Check sheet for the modelled part. Datum: model origin and axes. Units: mm. Face numbers are marked on the shaded views. Give positions to 0.01 mm unless a question says otherwise; leave off trailing zeros. Loops run counter-clockwise (first coordinate to the right, second up) from the corner with the lowest first, then second, coordinate; pieces in that order, holes last. Notation, with made-up numbers: M 14.25,83.5 L 54.25,83.5 A32 cw 54.25,117.5 Z; hole C 52,75 d4. An arc over 180 degrees is marked long. Write each question's results on one line, items separated by ' | '. Start each with the question number.
1. Material ranges on line 1 along X through (y, z) = (37, 0) (3 decimals); line 2 along Y through (x, z) = (-1.5, 22) (3 decimals); line 3 along Z through (x, y) = (-1.5, 36.5), recorded low to high.
2. Sectioned sample at C-C on y = 12. Record the cut outline in (x, z) (3 decimals).
3. Sectioned sample at A-A on z = 0. Record the cut outline in (x, y) (3 decimals), and give its area (3 significant figures).
4. Draft check along X on the marked faces 1, 2 and 3. Enter one of: pulls with the +X half, pulls with the -X half, needs draft (parallel to the pull), parting line crosses it, or undercut.
5. Go/stop test with flat-tipped pins: pin 1 (10 mm diameter, centred on x = -21.5, y = 41.5, fed in from +Z); pin 2 (1.5 mm diameter, centred on y = 16, z = 2.5, fed in from +X); pin 3 (12 mm diameter, centred on x = 23.5, z = -18.5, fed in from +Y); pin 4 (6 mm diameter, centred on y = 31, z = -3, fed in from -X). Record where each tip stops, or that it passes through.
6. Sectioned sample at B-B on x = 0. Record the cut outline in (y, z) (3 decimals), and give its area (3 significant figures).
```python
from build123d import *

# Parameters (mm, degrees)
SKETCH2_R           = 31.75
BOSS_EXTRUDE2_DEPTH = 50.8
SHELL1_T            = -3.175
FILLET2_R           = 2.54
CHAMFER1_SIZE       = 2.54


with BuildPart() as part:
    # Sketch2 → Boss-Extrude2 (new body)
    with BuildSketch(Plane(origin=(0, 0, 0), x_dir=(1, 0, 0), z_dir=(0, 1, 0))):
        with Locations(Location((0, 0, 0), (0, 0, 270))):
            Circle(SKETCH2_R)
    extrude(amount=BOSS_EXTRUDE2_DEPTH)

    # Shell1
    shell1_openings = [part.faces().sort_by_distance(p)[0] for p in [
        (0, 0, 0),
    ]]
    offset(amount=SHELL1_T, openings=shell1_openings, kind=Kind.INTERSECTION)

    # Fillet2
    fillet2_edges = [part.edges().sort_by_distance(p)[0] for p in [
        (0, 50.8, -31.75),
    ]]
    fillet(fillet2_edges, radius=FILLET2_R)

    # Chamfer1
    chamfer1_edges = [part.edges().sort_by_distance(p)[0] for p in [
        (0, 0, -28.575),
    ]]
    chamfer(chamfer1_edges, length=CHAMFER1_SIZE)


solid = part.part
```
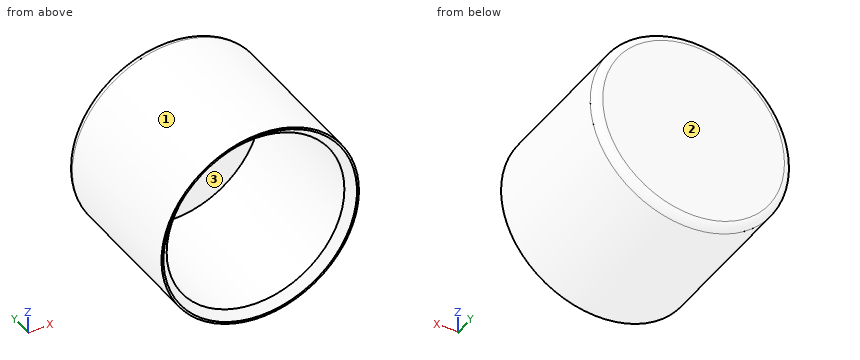
Output values:
1) line 1: -31.75 to -28.575, 28.575 to 31.75 | line 2: 47.625 to 50.8 | line 3: -31.71 to -28.54, 28.54 to 31.71
2) outline: C 0,0 d63.5; hole C 0,0 d57.15
3) outline: M -31.75,0 L -31.115,0 L -28.575,2.54 L -28.575,47.625 L 28.575,47.625 L 28.575,2.54 L 31.115,0 L 31.75,0 L 31.75,48.26 A2.54 ccw 29.21,50.8 L -29.21,50.8 A2.54 ccw -31.75,48.26 Z | area: 495 mm2
4) face 1: parting line crosses it | face 2: needs draft | face 3: undercut
5) pin 1: z = 27.13 | pin 2: x = 31.7 | pin 3: y = 50.8 | pin 4: x = -31.75
6) outline: M 0,-31.75 L 48.26,-31.75 A2.54 ccw 50.8,-29.21 L 50.8,29.21 A2.54 ccw 48.26,31.75 L 0,31.75 L 0,31.115 L 2.54,28.575 L 47.625,28.575 L 47.625,-28.575 L 2.54,-28.575 L 0,-31.115 Z | area: 495 mm2
